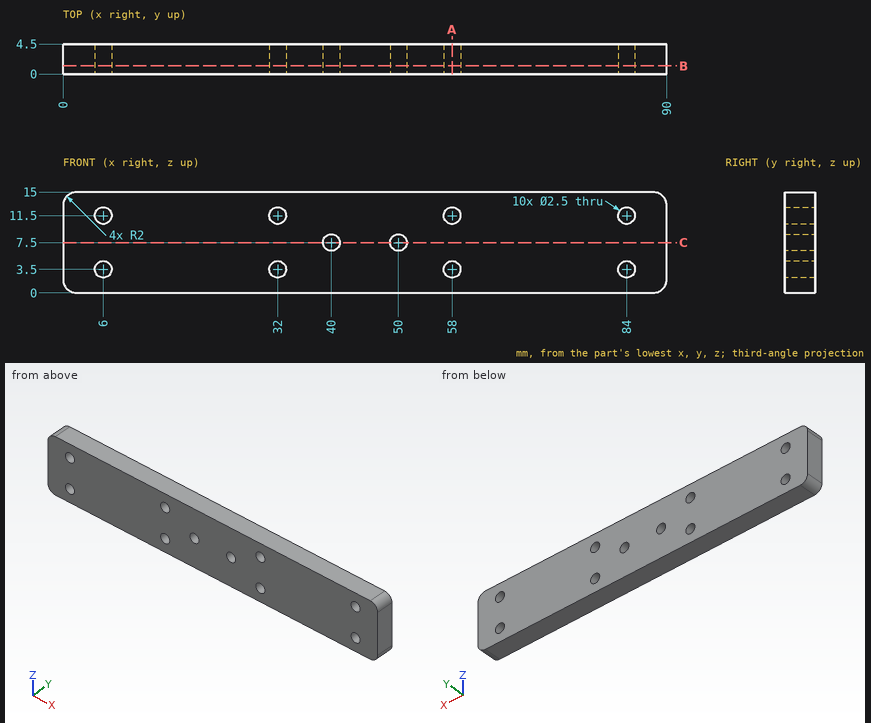
Can you work these out from the drawing? Everything is in mm from the part's minimum corner. Give positions to 0.01 mm unless a question says otherwise; leave off trailing zeros. Order: outer loops, then holes, each group sorted by start corner. A loop starts at its lowest first (then second) coordinate and runs counter-clockwise, first axis right, second up. Notation, with made-up numbers: (33.25, 26) -> (50.25, 26) arc R13 cw to (50.25, 35) -> close; hole circle Ø3 at (-39, -10.75). An arc over 180 degrees is marked (long way). Return JSON: item names as keys, results as strings.
1. Imagine slicing it at A-A on x = 58. List the corners of the cut face in (y, z) for me.
Answer list:
{"outline": "(0, 0) -> (4.5, 0) -> (4.5, 2.25) -> (0, 2.25) -> close; (0, 4.75) -> (4.5, 4.75) -> (4.5, 10.25) -> (0, 10.25) -> close; (0, 12.75) -> (4.5, 12.75) -> (4.5, 15) -> (0, 15) -> close"}
2. Imagine slicing it at C-C on z = 7.5. List the corners of the cut face in (x, y) for me, then the cut area to 4 significant figures.
Answer list:
{"outline": "(0, 0) -> (38.75, 0) -> (38.75, 4.5) -> (0, 4.5) -> close; (41.25, 0) -> (48.75, 0) -> (48.75, 4.5) -> (41.25, 4.5) -> close; (51.25, 0) -> (90, 0) -> (90, 4.5) -> (51.25, 4.5) -> close", "area": "382.5 mm2"}
3. For pin 1 Ø4 at (x, z) = (84, 11.5) entering from -Y; pin 2 Ø2 at (x, z) = (6, 3.5) entering from -Y, each with a flat end and sliding along its axis, tell me the tip position at first contact or that it passes through.
Answer list:
{"pin 1": "stops at y = 0", "pin 2": "passes through"}
4. Imagine slicing it at B-B on y = 1.25. Give the number of separate pieces and of enclosed holes in the cut face, then the cut area to 3 significant figures.
Answer list:
{"separate pieces": "1", "enclosed holes": "10", "area": "1,300 mm2"}
5. I need wall thicknesses on line 1 (X direction, y = 2, z = 3.5); line 2 (Z direction, x = 84, y = 1.95); line 3 (X direction, y = 1.8, z = 7.5). Which ranges of each line are inside material? Lowest first, please. Write a range as from..to.
Answer list:
{"line 1": "x = 0..4.75, 7.25..30.75, 33.25..56.75, 59.25..82.75, 85.25..90", "line 2": "z = 0..2.25, 4.75..10.25, 12.75..15", "line 3": "x = 0..38.75, 41.25..48.75, 51.25..90"}
